Geometry: final body of the model. Coordinates: model frame, mm. Give positions to 0.01 mm unless a question says otherwise; leave off trailing zeros. Order: outer loops, then holes, each group sorted by start corner. A loop starts at its lowest first (then second) coordinate and runs counter-clockwise, first axis right, second up. Notation, with made-up numbers: (17, -8.75) -> (23, -8.75) arc R17 ccw to (23, 11.25) -> close; hole circle Ø6 at (89, 88). An arc over 180 degrees is marked (long way). One line per item, written item: value. Start each with the question number.
```python
from build123d import *

# Parameters (mm, degrees)
SKETCH1_W          = 109
SKETCH1_H          = 3.18
SKETCH2_R          = 3.5
SKETCH2_W          = 23
SKETCH2_H          = 119
CUT_EXTRUDE1_DEPTH = 155.182075482


with BuildPart() as part:
    # Sketch1 → Revolve1 (revolve)
    with BuildSketch(Plane.XY, mode=Mode.PRIVATE) as revolve1_sk:
        with Locations((54.5, 1.59)):
            Rectangle(SKETCH1_W, SKETCH1_H)
    revolve(revolve1_sk.sketch.rotate(Axis((0, 4.511025306, 0), (0, 1, 0)), 90), axis=Axis((0, 4.511025306, 0), (0, 1, 0)))

    # Sketch2 → Cut-Extrude1 (cut, through all)
    with BuildSketch(Plane(origin=(0, 3.18, 0), x_dir=(1, 0, 0), z_dir=(0, 1, 0))):
        with Locations(Location((-50.5, 71.302237886, 0), (0, 0, 270))):
            Circle(SKETCH2_R)
        with Locations((-50.5, 0)):
            Rectangle(SKETCH2_W, SKETCH2_H)
    extrude(amount=-CUT_EXTRUDE1_DEPTH, mode=Mode.SUBTRACT)


solid = part.part
```
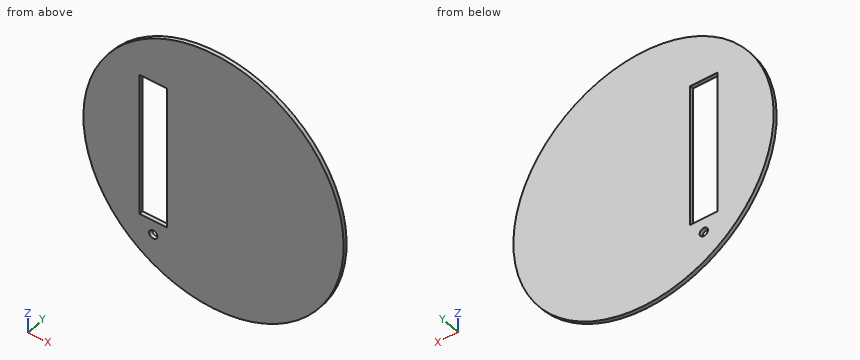
1. Pin query (flat end, axial travel): P1, Ø4, axis at x = -50.5, z = -71.3, coming from the +Y side; P2, Ø1.5, axis at y = 2, z = 59, coming from the +X side; P3, Ø1.6, axis at y = 2, z = 7.5, coming from the +X side; P4, Ø1, axis at x = -52, y = 2, coming from the -Z side. Return the tip coordinate at first contact, or that it passes through.
2. Cut plane C-C, the plane x = -50.5. Return loops of the section in (y, z).
3. Cut plane B-B, the plane y = 1.05. Return loops of the section in (x, z), then the cut area to 3 significant figures.
4. Cut plane D-D, the plane x = -21. Return loops of the section in (y, z).
5. Cut plane A-A, the plane z = 0. Return loops of the section in (x, y).
6. Material intervals for L1, parallel to X at y = 1.4, z = 0; L2, parallel to X at y = 1, z = -49; L3, parallel to Z at x = -40, y = 1.4, sorted ascending. Write a range as [from, to].
Answers follow:
1. P1: passes through
1. P2: stops at x = 92.13
1. P3: stops at x = 108.79
1. P4: stops at z = -96.07
2. outline: (0, -96.6) -> (3.18, -96.6) -> (3.18, -74.8) -> (0, -74.8) -> close; (0, -67.8) -> (3.18, -67.8) -> (3.18, -59.5) -> (0, -59.5) -> close; (0, 59.5) -> (3.18, 59.5) -> (3.18, 96.6) -> (0, 96.6) -> close
3. outline: circle Ø218 at (0, 0); hole (-62, -59.5) -> (-39, -59.5) -> (-39, 59.5) -> (-62, 59.5) -> close; hole circle Ø7 at (-50.5, -71.3)
3. area: 34,500 mm²
4. outline: (0, -106.96) -> (3.18, -106.96) -> (3.18, 106.96) -> (0, 106.96) -> close
5. outline: (-109, 0) -> (-62, 0) -> (-62, 3.18) -> (-109, 3.18) -> close; (-39, 0) -> (109, 0) -> (109, 3.18) -> (-39, 3.18) -> close
6. L1: x = [-109, -62], [-39, 109]
6. L2: x = [-97.37, -62], [-39, 97.37]
6. L3: z = [-101.4, -59.5], [59.5, 101.4]
